Part model, mm, in its own coordinate system. A direction names the side the tool comes from. Give positions to 0.01 mm unless a question says otherwise; leave off trailing zeros. Loops run counter-clockwise (first coordinate to the right, second up) from the corner with the lowest first, then second, coordinate; pieces in that order, holes last. Notation, with made-up numbers: M 16,3.5 L 68,3.5 A19 ccw 68,33.5 Z; hole C 10.5,-25 d2. An arc over 180 degrees is marked long. Put each result on its own line as item: value. Start each with the question number.
Autodesk Inventor part; units mm, degrees
ref_plane "YZ Plane" through (0, 0, 0) normal (1, 0, 0) x (0, 1, 0)
ref_plane "XZ Plane" through (0, 0, 0) normal (0, 1, 0) x (-1, 0, 0)
ref_plane "XY Plane" through (0, 0, 0) normal (0, 0, 1) x (1, 0, 0)
sketch "Base Sketch" plane through (0, 0, 0) normal (0, 1, 0) x (-1, 0, 0)
  line L0 (0, 0) -> (-26.9, 0)
  line L1 (-26.9, 0) -> (-26.9, -20)
  line L2 (-26.9, -20) -> (0, -20)
  line L3 (0, -20) -> (0, 0)
  line L4 (-14.2, -20) -> (-14.2, 0)
  line L5 (-10.6, -7.9793) -> (-7.1, -5.9585)
  line L6 (-7.1, -5.9585) -> (-3.6, -7.9793)
  line L7 (-3.6, -7.9793) -> (-3.6, -12.0207)
  line L8 (-3.6, -12.0207) -> (-7.1, -14.0415)
  line L9 (-7.1, -14.0415) -> (-10.6, -12.0207)
  line L10 (-10.6, -12.0207) -> (-10.6, -7.9793)
  point P0 (-20.55, -10)
  point P1 (-26.9, -10)
  point P2 (-7.1, -10)
  point P3 (0, -10)
  point P4 (-7.1, -10)
  dimension "d0" = 20
  dimension "d5" = 14.2
  dimension "d7" = 6.35
  dimension "d8" = 6.35
  dimension "d25" = 7.1
  dimension "d36" = 7
extrude "BasePlate" add sketch "Base Sketch" against normal blind 6 contours L3 L2 L4 L0 | L4 L2 L1 L0 | L5 L6 L7 L8 L9 L10
hole "Load Screw Hole" at (7.1, 0, -10) direction (0, -1, 0) diameter 4.2926 end through all
extrude "Top Section" add sketch "Base Sketch" along normal blind 6 contours L4 L2 L1 L0
sketch "Sketch2" plane through (0, 6, 0) normal (0, 1, 0) x (1, 0, 0)
  point P0 (20.55, 10)
hole "Extrusion Mount Screw" at (20.55, 6, -10) direction (0, -1, 0) diameter 4.2926 end through all counterbore diameter 8.001 counterbore depth 3.9878
chamfer "Chamfer" distance 1 angle 45 18 edges at (7.1, 0, -20) (14.2, 3, -20) (20.55, 6, -20) (26.9, 6, -10) (20.55, 6, 0) (14.2, 3, 0) (7.1, 0, 0) (0, -3, 0) (26.9, 0, 0) (26.9, 0, -20) (13.45, -6, -20) (26.9, -6, -10) (13.45, -6, 0) (0, -6, -10) (0, -3, -20) (0, 0, -10) (14.2, 6, -10) (20.55, 6, -14.0005)
extrude "Hex Nut Slot" cut sketch "Base Sketch" along normal blind 3.2 from surface at -6 contours L5 L6 L7 L8 L9 L10
thicken "Nut Fit Clearance" operation cut thickness 0.1 both sides no extend neighbours yes toward (-0.5, 0, 0.8660254) faces at (4.7667, -4.9333, -7.3057) (3.6, -4.9333, -10.6736) (5.9333, -4.9333, -13.3679) (9.4333, -4.9333, -12.6943) (10.6, -4.9333, -9.3264) (8.2667, -4.9333, -6.6321)
equation "\"d9\" = baseThickness"
equation "\"d22\" = chamferSize"
equation "\"baseThickness\" = 6"
equation "\"jawTravel\" = 3"
equation "\"M4_clearance_hole\" = 4.2"
equation "\"slotLength\" = M4_clearance_hole + jawTravel"
equation "\"chamferSize\" = 1"
properties material "ABS Plastic"
1) Band-saw the part on D-D on y = 1. Give the cut face in (x, z).
2) Band-saw the part on A-A on x = 20.55. Give the cut face in (y, z), then the cut area to 3 significant figures.
3) Pin check, flat tips, straight feed: pin 1 Ø2 at (x, z) = (6.5, -10.5) entering from -Y; pin 2 Ø6 at (x, z) = (6, -11) entering from +Y; pin 3 Ø1.5 at (y, z) = (3.5, -15) entering from -X. Stop position of each tip, or through.
4) Which spindle directions (+Z, -Z, +X, -X, +Y, -Y) get a long thin tool onto all of the face, cutting with end or side? Do faces 1 (the flat face through (10.7, -4, -10)), 2 (the cylindrical face through (16.584, 3.485, -10.521)), 3 (the flat face through (14.7, 2, -0.5)). Say none if no direction does.
5) Mould opens along X. For faces 4 (the flat face through (14.2, 2, -10)), 5 (the flat face through (13.3, -5.5, -19.5)), 6 (the flat face through (22, 2.012, -8)) say: +X half, -X half, draft (parallel to the pull), parting line (faces both ways), or undercut.
6) Band-saw the part on C-C on y = -1.5. Give the cut face in (x, z), then the cut area to 3 significant figures.
7) Band-saw the part on B-B on z = -10. State how many separate pieces and enclosed holes the cut face has, then the cut area to 3 significant figures.
8) Wall check: L1, parallel to X at y = -1.2, z = -10; L2, parallel to X at y = -3, z = -10; L3, parallel to X at y = 4.15, z = -10. Give the ranges that are in metal, low to high.
Evaluation:
1. outline: M 14.2,-19 L 15.2,-20 L 25.9,-20 L 26.9,-19 L 26.9,-1 L 25.9,0 L 15.2,0 L 14.2,-1 Z; hole C 20.55,-10 d4.29
2. outline: M -6,-19 L -5,-20 L 5,-20 L 6,-19 L 6,-15 L 5,-14 L 2.01,-14 L 2.01,-12.15 L -6,-12.15 Z; M -6,-7.85 L 2.01,-7.85 L 2.01,-6 L 5,-6 L 6,-5 L 6,-1 L 5,0 L -5,0 L -6,-1 Z
2. area: 171 mm2
3. pin 1: through
3. pin 2: y = 0
3. pin 3: x = 14.2
4. face 1: -Y
4. face 2: +Y
4. face 3: +Z, -X, +Y
5. face 4: -X half
5. face 5: draft
5. face 6: undercut
6. outline: M 0,-19 L 1,-20 L 25.9,-20 L 26.9,-19 L 26.9,-1 L 25.9,0 L 1,0 L 0,-1 Z; hole C 7.1,-10 d4.29; hole C 20.55,-10 d4.29
6. area: 507 mm2
7. separate pieces: 3
7. enclosed holes: 0
7. area: 133 mm2
8. L1: 0 to 4.95, 9.25 to 18.4, 22.7 to 26.9
8. L2: 0 to 3.5, 10.7 to 18.4, 22.7 to 26.9
8. L3: 14.2 to 16.55, 24.55 to 26.9
